Geometry check sheet. Reference: the model listing, model coordinates, mm. A direction names the side the tool comes from. Round coordinates to 2 decimals unless told otherwise and drop trailing zeros. Order: outer loops, then holes, each group sorted by start corner. A loop starts at its lowest first (then second) coordinate and runs counter-clockwise, first axis right, second up. Notation, with made-up numbers: (34, 14) - (73, 14) arc R32 ccw to (73, 53) - close; hole circle Ø5 at (14.5, 7.25). An arc over 180 degrees is marked (long way). One line per question, with ' | ' between items. Start each with the question number.
Q1. Mould release check, pull along Y, two halves, no side actions. Record for faces 1 (the face through (9.403, -34.662, 45.205)), 2 (the face through (-15.875, 57, 10)), 3 (the face through (-0.22, -61.99, 13.77)): +Y half, -Y half, draft (parallel to the pull), parting line (faces both ways), or undercut.
Q2. Gauge pin test, flat ends, axial feed: P1, Ø1.5, axis at x = -6.5, z = 5, coming from the +Y side; P2, Ø10, axis at x = 14, z = -49.5, coming from the -Y side; P3, Ø8, axis at y = 41, z = -17, coming from the -X side (3 decimals). Record the tip position at first contact, or that the pin passes through.
Q3. Material ranges on line 1 along Y through (x, z) = (9, 0); line 2 along Y through (x, z) = (-7, 0); line 3 along Y through (x, z) = (-12.5, -16), recorded low to high.
Q4. Tool access check on faces 4 (the face through (-3.175, 12, 23.2)), 5 (the face through (-17.462, 7, -12)), 6 (the face through (15.98, -17.36, 3.85)). Record the directions out of +Z, -Z, +X, -X, +Y, -Y that give a thin tool (end or side, any length) a straight path to the whole face; none if there is none.
Q5. Sectioned sample at A-A, the plane x = 11.5. Enter the section's corners in (y, z).
```python
from build123d import *


with BuildPart() as part:
    # Esboço1 → Revolução1 (revolve)
    with BuildSketch(Plane.XY, mode=Mode.PRIVATE) as revolu_o1_sk:
        with BuildLine():
            Line((-14.5288, 17.78), (-17.4625, 17.78))
            Line((-17.4625, 17.78), (-17.4625, 13.5001))
            Line((-17.4625, 13.5001), (17.4625, 13.5001))
            Line((17.4625, 13.5001), (17.4625, 17.78))
            Line((17.4625, 17.78), (14.5288, 17.78))
            Line((14.5288, 17.78), (14.5288, 19.05))
            Line((14.5288, 19.05), (8.971561034, 19.53619541))
            ThreePointArc((8.971561034, 19.53619541), (4.843288911, 21.572033925), (3.175, 25.862031743))
            Line((3.175, 25.862031743), (3.175, 50.601191018))
            ThreePointArc((3.175, 50.601191018), (4.843288911, 54.891188837), (8.971561034, 56.927027351))
            Line((8.971561034, 56.927027351), (15.875, 57.531))
            Line((15.875, 57.531), (15.875, 63.5))
            Line((15.875, 63.5), (-15.875, 63.5))
            Line((-15.875, 63.5), (-15.875, 57.531))
            Line((-15.875, 57.531), (-8.971561034, 56.927027351))
            ThreePointArc((-8.971561034, 56.927027351), (-4.843288911, 54.891188837), (-3.175, 50.601191018))
            Line((-3.175, 50.601191018), (-3.175, 25.862031743))
            ThreePointArc((-3.175, 25.862031743), (-4.843288911, 21.572033925), (-8.971561034, 19.53619541))
            Line((-8.971561034, 19.53619541), (-14.5288, 19.05))
            Line((-14.5288, 19.05), (-14.5288, 17.78))
        make_face()
    revolve(revolu_o1_sk.sketch.rotate(Axis((-17.4625, 0, 0), (1, 0, 0)), 270), axis=Axis((-17.4625, 0, 0), (1, 0, 0)))


solid = part.part
```
Determined:
1) face 1: undercut | face 2: draft | face 3: parting line
2) P1: stops at y = 63.36 | P2: stops at y = -45.3 | P3: stops at x = -3.175
3) line 1: y = -63.5 to -56.93, -19.53 to -13.5, 13.5 to 19.53, 56.93 to 63.5 | line 2: y = -63.5 to -56.43, -20.04 to -13.5, 13.5 to 20.04, 56.43 to 63.5 | line 3: y = -61.45 to -54.95, -10.66 to 10.66, 54.95 to 61.45
4) face 4: -X | face 5: +Z, -Z, -X, +Y, -Y | face 6: +X
5) outline: circle Ø127 at (0, 0); circle Ø38.63 at (0, 0); hole circle Ø114.3 at (0, 0); hole circle Ø27 at (0, 0)
